Model file for the job. Use its own axes, mm. Coordinates: 2 decimals unless noted, no trailing zeros. Order: outer loops, then holes, each group sorted by start corner. A loop starts at its lowest first (then second) coordinate and runs counter-clockwise, first axis right, second up. Notation, with made-up numbers: (52, 3) -> (91, 3) arc R28 cw to (91, 28) -> close; hole circle Ø9 at (-40, 79). An arc over 180 degrees is marked (long way). Write item = value, one per line. Start each with the question number.
Q1. Wall check: line 1 (Z direction, x = 203, y = 1.75); line 2 (X direction, y = 1.75, z = -62); line 3 (X direction, y = 3.5, z = -42). Give the ranges that are in metal, low to high. Write a range as from..to.
Q2. Cut at A-A, the plane x = 215.9. List the corners of the cut face in (y, z).
Q3. Mould opens along Z. For faces 1 (the face through (229.47, 3.22, -55.07)), 2 (the face through (213, 6.35, -116)) say: +Z half, -Z half, draft (parallel to the pull), parting line (faces both ways), or undercut.
Q4. Cut at B-B, the plane z = -50.8. List the corners of the cut face in (x, y).
from build123d import *

# Parameters (mm, degrees)
SKETCH2_W           = 431.8
SKETCH2_H           = 228.6
BOSS_EXTRUDE1_DEPTH = 6.35
SKETCH4_R           = 14.224
CUT_EXTRUDE1_DEPTH  = 6.35
SKETCH5_R           = 2.24967597
CUT_EXTRUDE2_DEPTH  = 25.4
SKETCH6_R           = 2.24967597
SKETCH6_R_2         = 2.249660739
SKETCH6_R_3         = 2.249660728
CUT_EXTRUDE3_DEPTH  = 25.4
SKETCH7_R           = 2.24967597
SKETCH7_R_2         = 2.249660728
CUT_EXTRUDE4_DEPTH  = 25.4


with BuildPart() as part:
    # Sketch2 → Boss-Extrude1 (new body)
    with BuildSketch(Plane(origin=(0, 0, 0), x_dir=(1, 0, 0), z_dir=(0, 1, 0))):
        with Locations((215.9, 114.3)):
            Rectangle(SKETCH2_W, SKETCH2_H)
    extrude(amount=BOSS_EXTRUDE1_DEPTH)

    # Sketch4 → Cut-Extrude1 (cut)
    with BuildSketch(Plane(origin=(0, 6.35, 0), x_dir=(1, 0, 0), z_dir=(0, 1, 0))):
        with Locations((215.9, 50.8)):
            Circle(SKETCH4_R)
    extrude(amount=-CUT_EXTRUDE1_DEPTH, mode=Mode.SUBTRACT)

    # Sketch5 → Cut-Extrude2 (cut)
    with BuildSketch(Plane(origin=(0, 0, 0), x_dir=(-1, 0, 0), z_dir=(0, -1, 0))):
        with Locations((-52.232812268, 111.081338493)):
            Circle(SKETCH5_R)
        with Locations((-52.232812268, 161.881338493)):
            Circle(SKETCH5_R)
    extrude(amount=-CUT_EXTRUDE2_DEPTH, mode=Mode.SUBTRACT)

    # Sketch6 → Cut-Extrude3 (cut)
    with BuildSketch(Plane(origin=(0, 0, 0), x_dir=(-1, 0, 0), z_dir=(0, -1, 0))):
        with Locations((-120.314890813, 111.081338493)):
            Circle(SKETCH6_R)
        with Locations((-120.314890813, 161.881338493)):
            Circle(SKETCH6_R)
        with Locations((-188.396969359, 111.081338493)):
            Circle(SKETCH6_R_2)
        with Locations((-188.396969359, 161.881338493)):
            Circle(SKETCH6_R_3)
    extrude(amount=-CUT_EXTRUDE3_DEPTH, mode=Mode.SUBTRACT)

    # Sketch7 → Cut-Extrude4 (cut)
    with BuildSketch(Plane(origin=(0, 0, 0), x_dir=(-1, 0, 0), z_dir=(0, -1, 0))):
        with Locations((-231.079047904, 111.081338493)):
            Circle(SKETCH7_R)
        with Locations((-231.079047904, 161.881338493)):
            Circle(SKETCH7_R_2)
        with Locations((-292.811126449, 111.081338493)):
            Circle(SKETCH7_R_2)
        with Locations((-292.811126449, 161.881338493)):
            Circle(SKETCH7_R_2)
        with Locations((-354.543204994, 111.081338493)):
            Circle(SKETCH7_R_2)
        with Locations((-354.543204994, 161.881338493)):
            Circle(SKETCH7_R_2)
    extrude(amount=-CUT_EXTRUDE4_DEPTH, mode=Mode.SUBTRACT)


solid = part.part
Here are the results:
q1.line_1 = -228.6..-56.79, -44.81..0
q1.line_2 = 0..207.13, 224.67..431.8
q1.line_3 = 0..204.72, 227.08..431.8
q2.outline = (0, -228.6) -> (6.35, -228.6) -> (6.35, -65.02) -> (0, -65.02) -> close; (0, -36.58) -> (6.35, -36.58) -> (6.35, 0) -> (0, 0) -> close
q3.face_1 = undercut
q3.face_2 = draft
q4.outline = (0, 0) -> (201.68, 0) -> (201.68, 6.35) -> (0, 6.35) -> close; (230.12, 0) -> (431.8, 0) -> (431.8, 6.35) -> (230.12, 6.35) -> close
